Here's how the part is built. I have some questions about the finished solid (model axes, mm). A direction names the side the tool comes from. Give positions to 0.01 mm unless a question says otherwise; leave off trailing zeros. Order: outer loops, then holes, each group sorted by start corner. A loop starts at its lowest first (then second) coordinate and runs counter-clockwise, first axis right, second up.
from build123d import *

# Parameters (mm, degrees)
FILLET4_R               = 3
CHAMFER1_SIZE2          = 0.393197641
CHAMFER1_SIZE           = 0.4
CUT_EXTRUDE1_DEPTH      = 14.804133806
CUT_EXTRUDE1_DEPTH_BACK = 8.0000001
FILLET5_R               = 0.4
FILLET6_R               = 0.8
FILLET7_R               = 0.2


with BuildPart() as part:
    # Sketch1 → Revolve1 (revolve)
    with BuildSketch(Plane.XY):
        Polygon((0, 1.825), (6.718918331, 1.825), (8.549810914, 1.3), (20.804133706, 1.5139), (20.804133706, 3.514204656), (8.813762579, 3.30491195), (7, 3.825), (7, 10), (4, 10), (4, 2.625), (0, 2.625), align=None)
    revolve(axis=Axis((0, 0, 0), (1, 0, 0)))

    # Fillet4
    fillet4_edges = [part.edges().sort_by_distance(p)[0] for p in [
        (8.549810914, -1.3, 0),
        (6.718918331, -1.825, 0),
    ]]
    fillet(fillet4_edges, radius=FILLET4_R)

    # Chamfer1
    chamfer1_edges = [part.edges().sort_by_distance(p)[0] for p in [
        (20.804133706, -3.514204656, 0),
    ]]
    chamfer(chamfer1_edges, length=CHAMFER1_SIZE, length2=CHAMFER1_SIZE2)

    # Sketch2 → Cut-Extrude1 (cut, two sides)
    with BuildSketch(Plane(origin=(7, 0, 0), x_dir=(0, 0, -1), z_dir=(1, 0, 0))) as cut_extrude1_sk:
        with BuildLine():
            Line((-10, 0), (-5, 8.660254038))
            ThreePointArc((-5, 8.660254038), (-8.660254038, 5), (-10, 0))
        make_face()
        with BuildLine():
            Line((-5, 8.660254038), (5, 8.660254038))
            ThreePointArc((5, 8.660254038), (0, 10), (-5, 8.660254038))
        make_face()
        with BuildLine():
            Line((5, 8.660254038), (10, 0))
            ThreePointArc((10, 0), (8.660254038, 5), (5, 8.660254038))
        make_face()
        with BuildLine():
            ThreePointArc((-10, 0), (-8.660254038, -5), (-5, -8.660254038))
            Line((-5, -8.660254038), (-10, 0))
        make_face()
        with BuildLine():
            ThreePointArc((-5, -8.660254038), (0, -10), (5, -8.660254038))
            Line((5, -8.660254038), (-5, -8.660254038))
        make_face()
        with BuildLine():
            ThreePointArc((5, -8.660254038), (8.660254038, -5), (10, 0))
            Line((10, 0), (5, -8.660254038))
        make_face()
    extrude(amount=CUT_EXTRUDE1_DEPTH, mode=Mode.SUBTRACT)
    extrude(cut_extrude1_sk.sketch, amount=-CUT_EXTRUDE1_DEPTH_BACK, mode=Mode.SUBTRACT)

    # Fillet5
    fillet5_edges = [part.edges().sort_by_distance(p)[0] for p in [
        (5.5, 8.660254038, 5),
        (5.5, 0, 10),
        (5.5, 0, -10),
        (5.5, 8.660254038, -5),
        (5.5, -8.660254038, 5),
        (5.5, -8.660254038, -5),
    ]]
    fillet(fillet5_edges, radius=FILLET5_R)

    # Fillet6
    fillet6_edges = [part.edges().sort_by_distance(p)[0] for p in [
        (7, -3.825, 0),
        (8.813762579, -3.30491195, 0),
    ]]
    fillet(fillet6_edges, radius=FILLET6_R)

    # Fillet7
    fillet7_edges = [part.edges().sort_by_distance(p)[0] for p in [
        (4, -2.625, 0),
    ]]
    fillet(fillet7_edges, radius=FILLET7_R)


solid = part.part
Q1. If we section it at B-B on x = 14.5: List the corners of the cut face in (y, z) for me.
Filled sheet:
outline: circle Ø6.81 at (0, 0); hole circle Ø2.81 at (0, 0)
Q2. If we section it at C-C on x = 12.25: List the corners of the cut face in (y, z) for me, plus the area to 3 significant figures.
Filled sheet:
outline: circle Ø6.73 at (0, 0); hole circle Ø2.73 at (0, 0)
area: 29.7 mm2
Q3. I'm going to push flat-ended pins straight in: P1, Ø6, axis at x = 18.5, y = -1.5, coming from the -Z side; P2, Ø5, axis at x = 11.5, y = 1.5, coming from the -Z side; P3, Ø3, axis at x = 14.5, y = -5, coming from the -Z side; P4, Ø1.5, axis at y = 1.5, z = 6.5, coming from the +X side. Where does each tip first touch, or does it pass through?
Filled sheet:
P1: stops at z = -3.51
P2: stops at z = -3.39
P3: passes through
P4: stops at x = 7
Q4. Thinking about a two-plate mould opening in Z: for faces 5 (the face through (14.98, 1.35, 0.42)), 6 (the face through (6, -8.66, 0)), 7 (the face through (5.521, -4.388, 7.467)), 8 (the face through (1.9, 2.5, 0.8)), which applies, released by +Z, released by -Z, zero draft, split by the parting line, or undercut?
Filled sheet:
face 5: undercut
face 6: zero draft
face 7: released by +Z
face 8: split by the parting line
Q5. I need wall thicknesses on L1, parallel to Z at x = 4.5, y = 0 (3 decimals); L2, parallel to Y at x = 4.25, z = 0 (3 decimals); L3, parallel to Z at x = 3.75, y = 0 (3 decimals). Which ranges of each line are inside material? Lowest first, please.
Filled sheet:
L1: z = -9.938 to -1.825, 1.825 to 9.938
L2: y = -8.66 to -1.825, 1.825 to 8.66
L3: z = -2.625 to -1.825, 1.825 to 2.625
Q6. For faces 1 (the face through (7, 2, -4.3)), 2 (the face through (3.19, 1.74, 0.55)), 3 (the face through (5.521, 4.272, 7.533)), 4 (the face through (14.592, -0.738, -3.325)), which set-ups out of +Z, -Z, +X, -X, +Y, -Y let a thin tool reach every point of the face, with its end or its side?
Filled sheet:
face 1: +X
face 2: -X
face 3: +Z, +X, -X, +Y
face 4: none
Q7. If we section it at A-A on x = 4.5: List the corners of the cut face in (y, z) for me (3 decimals), plus the area to 3 significant figures.
Filled sheet:
outline: (-8.66, -4.769) arc R0.4 ccw to (-8.46, -5.115) - (-0.2, -9.885) arc R0.4 ccw to (0.2, -9.885) - (8.46, -5.115) arc R0.4 ccw to (8.66, -4.769) - (8.66, 4.769) arc R0.4 ccw to (8.46, 5.115) - (0.2, 9.885) arc R0.4 ccw to (-0.2, 9.885) - (-8.46, 5.115) arc R0.4 ccw to (-8.66, 4.769) - close; hole circle Ø3.65 at (0, 0)
area: 249 mm2
